```python
from build123d import *

# Parameters (mm, degrees)
SKETCH1_W           = 19
SKETCH1_H           = 19
BOSS_EXTRUDE1_DEPTH = 7.6
CUT_EXTRUDE1_REACH  = 29.924
SKETCH2_W           = 6
SKETCH2_H           = 2.5
CUT_EXTRUDE2_REACH  = 29.924
SKETCH3_R           = 1.525
SKETCH4_R           = 5.05
CUT_EXTRUDE3_DEPTH  = 3.1
FILLET1_R           = 1
FILLET2_R           = 1
CUT_EXTRUDE4_REACH  = 29.244
SKETCH5_R           = 1.55


with BuildPart() as part:
    # Sketch1 → Boss-Extrude1 (new body)
    with BuildSketch(Plane(origin=(0, 0, 0), x_dir=(1, 0, 0), z_dir=(0, 1, 0))):
        with Locations((9.5, 9.5)):
            Rectangle(SKETCH1_W, SKETCH1_H)
    extrude(amount=BOSS_EXTRUDE1_DEPTH)

    # Sketch2 → Cut-Extrude1 (cut, up to next)
    with BuildSketch(Plane(origin=(19, 0, 0), x_dir=(0, 0, -1), z_dir=(1, 0, 0)), mode=Mode.PRIVATE) as cut_extrude1_sk1:
        with Locations((9.5, 5.35)):
            Rectangle(SKETCH2_W, SKETCH2_H)
    cut_extrude1_tool1 = extrude(cut_extrude1_sk1.sketch, amount=-CUT_EXTRUDE1_REACH, mode=Mode.PRIVATE) & part.part
    add(cut_extrude1_tool1.solids().sort_by_distance((19, 5.35, -9.5))[0], mode=Mode.SUBTRACT)

    # Sketch3 → Cut-Extrude2 (cut, up to next)
    with BuildSketch(Plane(origin=(0, 7.6, 0), x_dir=(1, 0, 0), z_dir=(0, 1, 0)), mode=Mode.PRIVATE) as cut_extrude2_sk1:
        with Locations(Location((3.25, 9.5, 0), (0, 0, 270))):
            Circle(SKETCH3_R)
    cut_extrude2_tool1 = extrude(cut_extrude2_sk1.sketch, amount=-CUT_EXTRUDE2_REACH, mode=Mode.PRIVATE) & part.part
    # Sketch3 → Cut-Extrude2 (cut, up to next)
    with BuildSketch(Plane(origin=(0, 7.6, 0), x_dir=(1, 0, 0), z_dir=(0, 1, 0)), mode=Mode.PRIVATE) as cut_extrude2_sk2:
        with Locations(Location((15.75, 9.5, 0), (0, 0, 270))):
            Circle(SKETCH3_R)
    cut_extrude2_tool2 = extrude(cut_extrude2_sk2.sketch, amount=-CUT_EXTRUDE2_REACH, mode=Mode.PRIVATE) & part.part
    add(cut_extrude2_tool1.solids().sort_by_distance((3.25, 7.6, -9.5))[0], mode=Mode.SUBTRACT)
    add(cut_extrude2_tool2.solids().sort_by_distance((15.75, 7.6, -9.5))[0], mode=Mode.SUBTRACT)

    # Sketch4 → Cut-Extrude3 (cut)
    with BuildSketch(Plane.XZ):
        with Locations(Location((9.5, -9.5, 0), (0, 0, 270))):
            Circle(SKETCH4_R)
    extrude(amount=-CUT_EXTRUDE3_DEPTH, mode=Mode.SUBTRACT)

    # Fillet1
    fillet1_edges = [part.edges().sort_by_distance(p)[0] for p in [
        (0, 3.8, -19),
        (19, 3.8, -19),
        (19, 3.8, 0),
        (0, 3.8, 0),
    ]]
    fillet(fillet1_edges, radius=FILLET1_R)

    # Fillet2
    fillet2_edges = [part.edges().sort_by_distance(p)[0] for p in [
        (9.5, 0, -4.45),
        (0, 0, -9.5),
        (9.5, 0, -19),
        (19, 0, -9.5),
        (9.5, 0, 0),
        (18.707106781, 0, -0.292893219),
        (0.292893219, 0, -0.292893219),
        (18.707106781, 0, -18.707106781),
        (0.292893219, 0, -18.707106781),
    ]]
    fillet(fillet2_edges, radius=FILLET2_R)

    # Sketch5 → Cut-Extrude4 (cut, up to next)
    with BuildSketch(Plane.XZ.offset(-3.1), mode=Mode.PRIVATE) as cut_extrude4_sk1:
        with Locations(Location((9.5, -9.5, 0), (0, 0, 270))):
            Circle(SKETCH5_R)
    cut_extrude4_tool1 = extrude(cut_extrude4_sk1.sketch, amount=-CUT_EXTRUDE4_REACH, mode=Mode.PRIVATE) & part.part
    add(cut_extrude4_tool1.solids().sort_by_distance((9.5, 3.1, -9.5))[0], mode=Mode.SUBTRACT)


solid = part.part
```
Build history of the part. All positions in model axes, mm. A direction names the side the tool comes from. Give positions to 0.01 mm unless a question says otherwise; leave off trailing zeros. Loops run counter-clockwise (first coordinate to the right, second up) from the corner with the lowest first, then second, coordinate; pieces in that order, holes last.
Item 1: Pull direction Y, two halves, no side cores. Call faces 1 (the face through (9, 4, 0)), 2 (the face through (8, 3.1, -8)), 3 (the face through (10, 6.6, -9)): released by +Y, released by -Y, zero draft, split by the parting line, or undercut.
Answers follow:
face 1: zero draft
face 2: released by -Y
face 3: undercut
Item 2: Drill centre lines: line 1 (X direction, y = 7.25, z = -9.5) (3 decimals); line 2 (Y direction, x = 7, z = -11.25); line 3 (Z direction, x = 1.5, y = 4.75). Where is each one in solid material? Low to high.
Answers follow:
line 1: x = 0 to 1.725, 4.775 to 14.225, 17.275 to 19
line 2: y = 3.1 to 4.1, 6.6 to 7.6
line 3: z = -19 to -12.5, -6.5 to 0
Item 3: Slice it at D-D, the plane x = 1.5. List the corners of the cut face in (y, z).
Answers follow:
outline: (0, -18) arc R1 ccw to (1, -19) - (7.6, -19) - (7.6, 0) - (1, 0) arc R1 ccw to (0, -1) - close; hole (4.1, -12.5) - (6.6, -12.5) - (6.6, -6.5) - (4.1, -6.5) - close
Item 4: Flat gauge pins, fed straight in: pin 1 (4 mm diameter, centred on x = 8, z = -12, fed in from -Y); pin 2 (2.5 mm diameter, centred on x = 9.5, z = -9.5, fed in from -Y). Where does each tip first touch, or does it go through?
Answers follow:
pin 1: stops at y = 3.1
pin 2: stops at y = 6.6
Item 5: Slice it at B-B, the plane y = 2.5. List the corners of the cut face in (x, z).
Answers follow:
outline: (0, -18) arc R1 ccw to (1, -19) - (18, -19) arc R1 ccw to (19, -18) - (19, -1) arc R1 ccw to (18, 0) - (1, 0) arc R1 ccw to (0, -1) - close; hole circle Ø10.1 at (9.5, -9.5)
Item 6: Which spindle directions (+Z, -Z, +X, -X, +Y, -Y) get a long thin tool onto all of the face, cutting with end or side? Do faces 4 (the face through (8.56, 3.59, -8.27)), 5 (the face through (9.381, 0.301, -0.285)), 6 (the face through (14.397, 7.107, -8.796)), 7 (the face through (10, 5, -12.5)), 8 (the face through (18.699, 4.346, -18.715)). Say none if no direction does.
Answers follow:
face 4: -Y
face 5: +Z, +X, -X, -Y
face 6: +Y
face 7: +X, -X
face 8: -Z, +X, +Y, -Y
Item 7: Slice it at A-A, the plane z = -9.5. List the corners of the cut face in (x, y) (3 decimals), and give its area (3 significant figures).
Answers follow:
outline: (0, 1) arc R1 ccw to (1, 0) - (3.45, 0) arc R1 ccw to (4.45, 1) - (4.45, 3.1) - (7.95, 3.1) - (7.95, 4.1) - (0, 4.1) - close; (0, 6.6) - (1.725, 6.6) - (1.725, 7.6) - (0, 7.6) - close; (4.775, 6.6) - (14.225, 6.6) - (14.225, 7.6) - (4.775, 7.6) - close; (11.05, 3.1) - (14.55, 3.1) - (14.55, 1) arc R1 ccw to (15.55, 0) - (18, 0) arc R1 ccw to (19, 1) - (19, 4.1) - (11.05, 4.1) - close; (17.275, 6.6) - (19, 6.6) - (19, 7.6) - (17.275, 7.6) - close
area: 55.5 mm2
Item 8: Slice it at C-C, the plane y = 7. List the corners of the cut face in (x, z) (3 decimals).
Answers follow:
outline: (0, -18) arc R1 ccw to (1, -19) - (18, -19) arc R1 ccw to (19, -18) - (19, -1) arc R1 ccw to (18, 0) - (1, 0) arc R1 ccw to (0, -1) - close; hole circle Ø3.05 at (3.25, -9.5); hole circle Ø3.05 at (15.75, -9.5)
